```python
from build123d import *

# Parameters (mm, degrees)
BOSS_EXTRUDE2_DEPTH      = 34.479411165
BOSS_EXTRUDE2_DEPTH_BACK = 0.1
SKETCH4_W                = 120
SKETCH4_H                = 185
SKETCH7_W                = 88.965159514
SKETCH7_H                = 168.79001582
CUT_EXTRUDE1_DEPTH       = 32
SKETCH8_W                = 38.11885966
SKETCH8_H                = 26.011926246
CUT_EXTRUDE2_DEPTH       = 32
SKETCH12_W               = 12.33668545
SKETCH12_H               = 28.735157877
SKETCH12_W_2             = 13.054734016
CUT_EXTRUDE10_DEPTH      = 169
CUT_EXTRUDE11_DEPTH      = 156.38687137
CUT_EXTRUDE11_DEPTH_BACK = 120
SKETCH14_W               = 7.893435911
SKETCH14_H               = 7.893435911
SKETCH14_W_2             = 7.893435912
CUT_EXTRUDE13_DEPTH      = 120
SKETCH16_W               = 16.234881207
SKETCH16_H               = 30.372514135
CUT_EXTRUDE15_DEPTH      = 30


with BuildPart() as part:
    # Sketch4 → Boss-Extrude2 (new, two sides: drawn at the far end of the back side and taken through both)
    with BuildSketch(Plane.XY.offset(-BOSS_EXTRUDE2_DEPTH_BACK)):
        Rectangle(SKETCH4_W, SKETCH4_H)
    extrude(amount=BOSS_EXTRUDE2_DEPTH + BOSS_EXTRUDE2_DEPTH_BACK)

    # Sketch7 → Cut-Extrude1 (cut)
    with BuildSketch(Plane(origin=(0, 0, -0.1), x_dir=(-1, 0, 0), z_dir=(0, 0, -1))):
        with Locations((0.239153655, 8.10499209)):
            Rectangle(SKETCH7_W, SKETCH7_H)
    extrude(amount=-CUT_EXTRUDE1_DEPTH, mode=Mode.SUBTRACT)

    # Sketch8 → Cut-Extrude2 (cut)
    with BuildSketch(Plane(origin=(0, -76.29001582, 0), x_dir=(1, 0, 0), z_dir=(0, 1, 0))):
        with Locations((0.239741256, -16.26190688)):
            Rectangle(SKETCH8_W, SKETCH8_H)
    extrude(amount=-CUT_EXTRUDE2_DEPTH, mode=Mode.SUBTRACT)

    # Sketch12 → Cut-Extrude10 (cut)
    with BuildSketch(Plane(origin=(0, 92.5, 0), x_dir=(1, 0, 0), z_dir=(0, 1, 0))):
        with Locations((-50.890076137, -17.532421062)):
            Rectangle(SKETCH12_W, SKETCH12_H)
        with Locations((50.77079311, -17.532421062)):
            Rectangle(SKETCH12_W_2, SKETCH12_H)
    extrude(amount=-CUT_EXTRUDE10_DEPTH, mode=Mode.SUBTRACT)

    # Sketch13 → Cut-Extrude11 (cut, two sides: drawn at the far end of the back side and taken through both)
    with BuildSketch(Plane(origin=(60, 0, 0), x_dir=(0, 0, -1), z_dir=(1, 0, 0)).offset(-CUT_EXTRUDE11_DEPTH_BACK)):
        Polygon((-247.325576021, 407.948170503), (-27.952099996, 92.5), (-11.689651482, 69.115406181), (0.1, 69.115406181), (384.329450013, 69.115406181), (747.583784475, 746.297338547), (115.928758441, 1085.130102868), align=None)
    extrude(amount=CUT_EXTRUDE11_DEPTH + CUT_EXTRUDE11_DEPTH_BACK, mode=Mode.SUBTRACT)

    # Sketch14 → Cut-Extrude13 (cut)
    with BuildSketch(Plane(origin=(0, 0, 31.9), x_dir=(-1, 0, 0), z_dir=(0, 0, -1))):
        with Locations((-32.983285774, 84.758555925)):
            Rectangle(SKETCH14_W, SKETCH14_H)
        with Locations((31.155523105, 84.758555925)):
            Rectangle(SKETCH14_W_2, SKETCH14_H)
    extrude(amount=-CUT_EXTRUDE13_DEPTH, mode=Mode.SUBTRACT)

    # Sketch16 → Cut-Extrude15 (cut)
    with BuildSketch(Plane.XY.offset(34.479411165)):
        with Locations((51.882559396, 22.360866706)):
            Rectangle(SKETCH16_W, SKETCH16_H)
    extrude(amount=-CUT_EXTRUDE15_DEPTH, mode=Mode.SUBTRACT)


solid = part.part
```
Check sheet for the modelled part. Datum: model origin and axes. Units: mm. A direction names the side the tool comes from. Coordinates: 2 decimals unless noted, no trailing zeros. Order: outer loops, then holes, each group sorted by start corner. A loop starts at its lowest first (then second) coordinate and runs counter-clockwise, first axis right, second up. Notation, with made-up numbers: (-38, 88) -> (14, 88) arc R22 cw to (14, 97) -> close; hole circle Ø4 at (8.25, -33). An arc over 180 degrees is marked (long way). Write each question's results on one line, items separated by ' | '. Start each with the question number.
1) Section check D-D (x = -41). Enter the section's corners in (y, z), and give its area (3 significant figures).
2) Draft check along Y on faces 6 (the face through (-1, 9, 31.9)), 7 (the face through (58, 37.547, 24)), 8 (the face through (58, 7.175, 24)), 9 (the face through (-51, -76.5, 17)). Enter one of: pulls with the +Y half, pulls with the -Y half, needs draft (parallel to the pull), parting line crosses it, or undercut.
3) Material ranges on line 1 along Z through (x, y) = (-45.5, -18); line 2 along X through (y, z) = (80, 26); line 3 along X through (y, z) = (-84.5, 22), recorded low to high.
4) Depth check by flat-ended pin: pin 1 (1.5 mm diameter, centred on x = 1, y = 13, fed in from -Z); pin 2 (13 mm diameter, centred on x = -50, z = 4, fed in from +Y); pin 3 (6 mm diameter, centred on x = -32.5, z = 13, fed in from +Y). Enter the tip coordinate at first touch or a pass-through.
5) Section check C-C (z = 6.5). Enter the section's corners in (x, y).
6) Section check B-B (x = -8). Enter the section's corners in (y, z).
7) Section check A-A (y = 9). Enter the section's corners in (x, z), and give its area (3 significant figures).
8) Set-up check for faces 1 (the face through (19.299, -84, 16)), 2 (the face through (-56, 69.115, 2)), 3 (the face through (-1, -92.5, 32)), 4 (the face through (-51, -3, 3.165)), 5 (the face through (0, -76.29, 30)): record each of +Z, -Z, +X, -X, +Y, -Y from which the full face is reachable in a straight line by a thin tool's end or side.
Checked values:
1) outline: (-92.5, -0.1) -> (-76.29, -0.1) -> (-76.29, 31.9) -> (92.5, 31.9) -> (92.5, 34.48) -> (-92.5, 34.48) -> close | area: 996 mm²
2) face 6: needs draft | face 7: undercut | face 8: undercut | face 9: pulls with the +Y half
3) line 1: -0.1 to 3.16, 31.9 to 34.48 | line 2: -60 to -57.06, 57.3 to 60 | line 3: -60 to -18.82, 19.3 to 60
4) pin 1: z = 31.9 | pin 2: y = 69.12 | pin 3: y = -76.29
5) outline: (-60, -92.5) -> (-18.82, -92.5) -> (-18.82, -76.29) -> (-44.72, -76.29) -> (-44.72, -76.5) -> (-57.06, -76.5) -> (-57.06, 69.12) -> (-60, 69.12) -> close; (19.3, -92.5) -> (60, -92.5) -> (60, 7.17) -> (57.3, 7.17) -> (57.3, -76.5) -> (44.24, -76.5) -> (44.24, -76.29) -> (19.3, -76.29) -> close; (57.3, 37.55) -> (60, 37.55) -> (60, 69.12) -> (57.3, 69.12) -> close
6) outline: (-92.5, -0.1) -> (-76.29, -0.1) -> (-76.29, 3.26) -> (-92.5, 3.26) -> close; (-92.5, 29.27) -> (-76.29, 29.27) -> (-76.29, 31.9) -> (92.5, 31.9) -> (92.5, 34.48) -> (-92.5, 34.48) -> close
7) outline: (-60, -0.1) -> (-44.72, -0.1) -> (-44.72, 3.16) -> (-57.06, 3.16) -> (-57.06, 31.9) -> (43.77, 31.9) -> (43.77, 34.48) -> (-60, 34.48) -> close; (44.24, -0.1) -> (60, -0.1) -> (60, 4.48) -> (57.3, 4.48) -> (57.3, 3.16) -> (44.24, 3.16) -> close | area: 457 mm²
8) face 1: +Y, -Y | face 2: -Z, +X, -X, +Y | face 3: +Z, -Z, +X, -X, -Y | face 4: +Y | face 5: -Z, +Y
